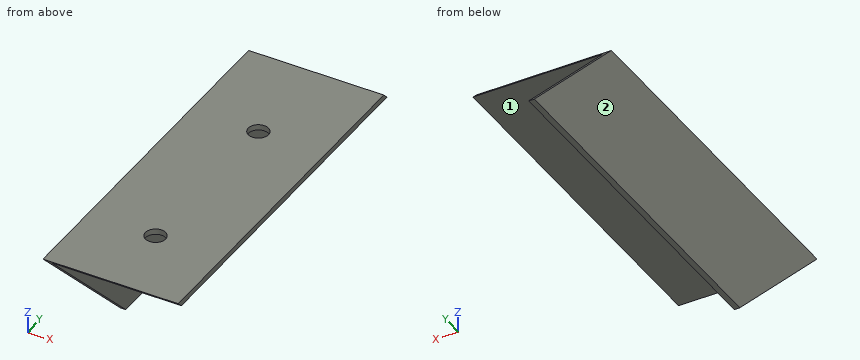
from build123d import *

# Parameters (mm, degrees)
F1_DEPTH = 220
F3_DEPTH = 60.001
F4_R     = 4.5
F5_DEPTH = 60.001


with BuildPart() as f1:
    # F0 (on Front) → F1 (new body)
    with BuildSketch(Plane.XZ):
        Polygon((60, 0), (0, 0), (0, -60), (2.5, -60), (2.5, -2.5), (60, -2.5), align=None)
    extrude(amount=F1_DEPTH)

    # F2 (on face) → F3 (cut, through all)
    with BuildSketch(Plane(origin=(0, 0, 0), x_dir=(0, -1, 0), z_dir=(-1, 0, 0))):
        Polygon((0, 0), (0, -60), (60, 0), align=None)
        Polygon((220, -60), (220, 0), (160, -60), align=None)
    extrude(amount=-F3_DEPTH, mode=Mode.SUBTRACT)

    # F4 (on face) → F5 (cut, through all)
    with BuildSketch(Plane.XY):
        with Locations((30, -105)):
            Circle(F4_R)
        with Locations((30, -185)):
            Circle(F4_R)
    extrude(amount=-F5_DEPTH, mode=Mode.SUBTRACT)


solid = f1.part
Could you check a few things on this model? Use its own coordinates, in mm. Face numbers are marked on the shaded views. A direction names the side the tool comes from. Coordinates: 2 decimals unless noted, no trailing zeros. Write each loop counter-clockwise with the first axis right and the second up, starting at its lowest first coordinate (ties: lowest second). Pieces come first, ordered by that corner, then holes. Notation, with made-up numbers: (1, -15) - (36, -15) arc R19 ccw to (36, -11) - close; hole circle Ø10 at (39, 83). An arc over 180 degrees is marked (long way). Put each result on its own line as item: value. Start each with the question number.
Q1. Please list where these lines run through material, in increasing order: L1, parallel to Y at x = 30, z = -1.9; L2, parallel to Y at x = 30, z = -1.7; L3, parallel to Z at x = 36, y = -101.
Q2. I'm going to push flat-ended pins straight in: P1, Ø5.5, axis at x = 30, y = -185, coming from the -Z side; P2, Ø1.5, axis at y = -144.5, z = -9.5, coming from the +X side; P3, Ø1.5, axis at x = 20, y = -150.5, coming from the -Z side. Where does each tip first touch, or does it pass through?
Q3. I want a section at D-D on z = -17.5. Write out the boundary of the cut face in (x, y).
Q4. I want a section at B-B on x = 30. Write out the boundary of the cut face in (y, z).
Q5. I want a section at A-A on y = -105. Write out the boundary of the cut face in (x, z), plus the area to 3 significant figures.
Q6. Which directions (+Z, -Z, +X, -X, +Y, -Y) give clear straight access to the entire face, cutting with the end or side of a thin tool? Please do the marked faces 1 and 2.
Q7. I want a section at C-C on y = -185. Write out the boundary of the cut face in (x, z), plus the area to 3 significant figures.
Checks:
1. L1: -218.1 to -189.5, -180.5 to -109.5, -100.5 to -58.1
1. L2: -218.3 to -189.5, -180.5 to -109.5, -100.5 to -58.3
1. L3: -2.5 to 0
2. P1: through
2. P2: x = 2.5
2. P3: z = -2.5
3. outline: (0, -202.5) - (2.5, -202.5) - (2.5, -42.5) - (0, -42.5) - close
4. outline: (-220, 0) - (-217.5, -2.5) - (-189.5, -2.5) - (-189.5, 0) - close; (-180.5, -2.5) - (-109.5, -2.5) - (-109.5, 0) - (-180.5, 0) - close; (-100.5, -2.5) - (-57.5, -2.5) - (-60, 0) - (-100.5, 0) - close
5. outline: (0, -60) - (2.5, -60) - (2.5, -2.5) - (25.5, -2.5) - (25.5, 0) - (0, 0) - close; (34.5, -2.5) - (60, -2.5) - (60, 0) - (34.5, 0) - close
5. area: 271 mm²
6. face 1: -Z, +X, +Y, -Y
6. face 2: +Z, -Z, -X, +Y, -Y
7. outline: (0, -35) - (2.5, -35) - (2.5, -2.5) - (25.5, -2.5) - (25.5, 0) - (0, 0) - close; (34.5, -2.5) - (60, -2.5) - (60, 0) - (34.5, 0) - close
7. area: 209 mm²
